For this review, take the finished solid that the model builds, in its own axes (mm). A direction names the side the tool comes from. Round coordinates to 2 decimals unless told otherwise and drop trailing zeros. Order: outer loops, then holes, each group sorted by start corner. A loop starts at its lowest first (then second) coordinate and runs counter-clockwise, first axis right, second up.
from build123d import *

# Parameters (mm, degrees)
BOSS_EXTRUDE1_DEPTH              = 342.9
BOSS_EXTRUDE1_DEPTH_BACK         = 342.9
SKETCH3_W                        = 50.8
SKETCH3_H                        = 25.4
SKETCH3_W_2                      = 44.45
SKETCH3_H_2                      = 19.05
F_1_4_0_25_DIAMETER_HOLE3_D      = 6.35
F_1_4_0_25_DIAMETER_HOLE4_D      = 6.35
F_1_4_0_25_DIAMETER_HOLE5_D      = 6.35
F_1_4_0_25_DIAMETER_HOLE6_D      = 6.35
F_1_4_0_25_DIAMETER_HOLE7_D      = 6.35
F_1_4_0_25_DIAMETER_HOLE8_D      = 6.35
F_13_64_0_20313_DIAMETER_HOLE1_D = 5.159502
F_1_2_0_5_DIAMETER_HOLE1_D       = 12.7
F_1_2_0_5_DIAMETER_HOLE1_DEPTH   = 6.35
F_1_2_0_5_DIAMETER_HOLE1_TIP     = 3.815464931


with BuildPart() as part:
    # Sketch3 → Boss-Extrude1 (new, two sides: drawn at the far end of the back side and taken through both)
    with BuildSketch(Plane.XY.offset(-BOSS_EXTRUDE1_DEPTH_BACK)):
        Rectangle(SKETCH3_W, SKETCH3_H)
        Rectangle(SKETCH3_W_2, SKETCH3_H_2, mode=Mode.SUBTRACT)
    extrude(amount=BOSS_EXTRUDE1_DEPTH + BOSS_EXTRUDE1_DEPTH_BACK)

    # 1/4 (0.25) Diameter Hole3 (through all)
    with Locations(Plane.ZY.offset(25.4)):
        with Locations((-330.2, 0)):
            Hole(F_1_4_0_25_DIAMETER_HOLE3_D / 2)

    # 1/4 (0.25) Diameter Hole4 (through all)
    with Locations(Plane.ZY.offset(25.4)):
        with Locations((304.8, 0), (330.2, 0)):
            Hole(F_1_4_0_25_DIAMETER_HOLE4_D / 2)

    # 1/4 (0.25) Diameter Hole5 (through all)
    with Locations(Plane(origin=(25.4, 0, 0), x_dir=(0, 0, -1), z_dir=(1, 0, 0))):
        with Locations((304.8, 0), (279.4, 0)):
            Hole(F_1_4_0_25_DIAMETER_HOLE5_D / 2)

    # 1/4 (0.25) Diameter Hole6 (through all)
    with Locations(Plane(origin=(25.4, 0, 0), x_dir=(0, 0, -1), z_dir=(1, 0, 0))):
        with Locations((228.6, 0), (254, 0)):
            Hole(F_1_4_0_25_DIAMETER_HOLE6_D / 2)

    # 1/4 (0.25) Diameter Hole7 (through all)
    with Locations(Plane(origin=(25.4, 0, 0), x_dir=(0, 0, -1), z_dir=(1, 0, 0))):
        with Locations((-203.2, 0), (-228.6, 0)):
            Hole(F_1_4_0_25_DIAMETER_HOLE7_D / 2)

    # 1/4 (0.25) Diameter Hole8 (through all)
    with Locations(Plane(origin=(25.4, 0, 0), x_dir=(0, 0, -1), z_dir=(1, 0, 0))):
        with Locations((-279.4, 0), (-254, 0)):
            Hole(F_1_4_0_25_DIAMETER_HOLE8_D / 2)

    # 13/64 (0.20313) Diameter Hole1 (through all)
    with Locations(Plane(origin=(25.4, 0, 0), x_dir=(0, 0, -1), z_dir=(1, 0, 0))):
        with Locations((-152.4, 0), (177.8, 0)):
            Hole(F_13_64_0_20313_DIAMETER_HOLE1_D / 2)

    # 1/2 (0.5) Diameter Hole1
    with Locations(Plane.ZY.offset(25.4)):
        with Locations((-591.301639708, -480.802221962), (-103.1875, 0), (77.7875, 0), (103.1875, 0), (-128.5875, 0)):
            Hole(F_1_2_0_5_DIAMETER_HOLE1_D / 2, depth=F_1_2_0_5_DIAMETER_HOLE1_DEPTH)
            with Locations((0, 0, -(F_1_2_0_5_DIAMETER_HOLE1_DEPTH + F_1_2_0_5_DIAMETER_HOLE1_TIP / 2))):  # 118° drill point
                Cone(0, F_1_2_0_5_DIAMETER_HOLE1_D / 2, F_1_2_0_5_DIAMETER_HOLE1_TIP, mode=Mode.SUBTRACT)


solid = part.part
(1) Wall thickness on L1, parallel to Y at x = -20.5, z = 176 (3 decimals); L2, parallel to X at y = -1, z = -33 (3 decimals); L3, parallel to Y at x = 23, z = 203: over which ranges is each line inside the solid? List them lowest first.
(2) Add section A-A on z = -153. Give the boundary of the cut face in (x, y) (3 decimals).
(3) Tool access review of faces 4 (the face through (0, 9.525, -5)), 5 (the face through (-23.79, 0.279, -122.244)), 6 (the face through (25.4, 0, -5)): name each direction out of +Z, -Z, +X, -X, +Y, -Y from which nothing blocks a thin tool from reaching the whole face with its end or side.
(4) Add section B-B on x = -11. Give the boundary of the cut face in (y, z) (3 decimals).
(5) Draft analysis for pull direction X (two halves, no side actions). For faces 1 (the face through (-23.79, 0.28, 84.13)), 2 (the face through (-25.4, 0, -5)), 3 (the face through (0, -9.525, -5)), state which applies: pulls with the +X half, pulls with the -X half, needs draft (parallel to the pull), parting line crosses it, or undercut.
(6) Clearance check with flat-ended pins moving along their axes: P1, Ø6, axis at y = 0, z = 152.4, coming from the +X side; P2, Ø5.5, axis at y = 0, z = 228.6, coming from the +X side; P3, Ø11.5, axis at y = 0, z = 77.79, coming from the -X side (3 decimals). State where each tip first meets the part, or that it passes through.
Here are the results:
1. L1: y = -12.7 to -9.525, 9.525 to 12.7
1. L2: x = -25.4 to -22.225, 22.225 to 25.4
1. L3: y = -12.7 to -3.17, 3.17 to 12.7
2. outline: (-25.4, -12.7) - (25.4, -12.7) - (25.4, 12.7) - (-25.4, 12.7) - close; hole (-22.225, -9.525) - (22.225, -9.525) - (22.225, 9.525) - (-22.225, 9.525) - close
3. face 4: +Z, -Z
3. face 5: -X
3. face 6: +Z, -Z, +X, +Y, -Y
4. outline: (-12.7, -342.9) - (-9.525, -342.9) - (-9.525, 342.9) - (-12.7, 342.9) - close; (9.525, -342.9) - (12.7, -342.9) - (12.7, 342.9) - (9.525, 342.9) - close
5. face 1: needs draft
5. face 2: pulls with the -X half
5. face 3: undercut
6. P1: stops at x = 25.4
6. P2: passes through
6. P3: stops at x = 22.225
